Check sheet for the modelled part. Datum: model origin and axes. Units: mm. Coordinates: 2 decimals unless noted, no trailing zeros. Loops run counter-clockwise (first coordinate to the right, second up) from the corner with the lowest first, then second, coordinate; pieces in that order, holes last. Notation, with made-up numbers: M 84.25,73.5 L 104.25,73.5 A26 ccw 104.25,93.5 Z; hole C 23.5,-14 d9. An arc over 180 degrees is marked long. Use CSV: the item, a comma, the result in double quotes. Start each with the question number.
(1) Go/stop test with flat-tipped pins: pin 1 Ø1 at (x, z) = (-7, 1.5) entering from -Y; pin 2 Ø4 at (x, y) = (6.5, 0) entering from -Z; pin 3 Ø1 at (x, z) = (26.5, 1.5) entering from -Y. Record where each tip stops, or that it passes through.
(2) Section check C-C on x = -16.5. Record the cut outline in (y, z), and give its area (3 significant figures).
(3) Section check A-A on x = 6.5. Record the cut outline in (y, z) (3 decimals).
(4) Section check D-D on y = -27. Record the cut outline in (x, z), and give its area (3 significant figures).
(5) Section check B-B on z = 1.7. Record the cut outline in (x, y) (3 decimals), and give its area (3 significant figures).
(6) Scan lines: line 1 (Y direction, x = 6.5, z = 1.25) (3 decimals); line 2 (Y direction, x = 51, z = 0.3); line 3 (Y direction, x = -6.5, z = 1). Record each from-to range of solid material in increasing order.
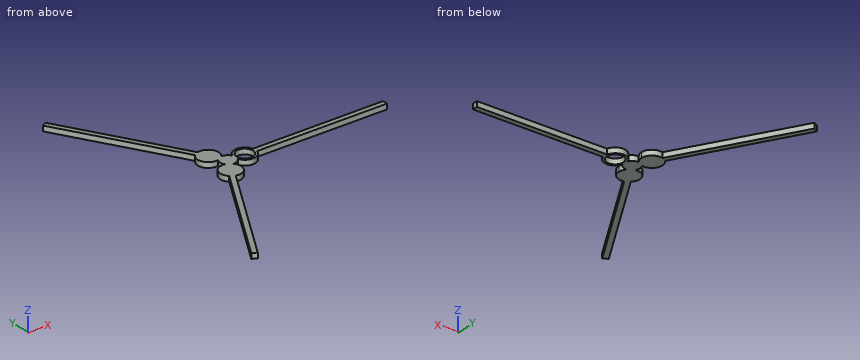
from build123d import *

# Parameters (mm, degrees)
F1_DEPTH = 2
F2_R     = 3.175
F3_DEPTH = 25


with BuildPart() as f1:
    # F0 (on Top) → F1 (new body)
    with BuildSketch(Plane.XY):
        with BuildLine():
            ThreePointArc((2.7115384615, -1.2835728151), (2.9269963601, -0.6577935145), (3, 0))
            ThreePointArc((3, 0), (2.9269963601, 0.6577935145), (2.7115384615, 1.2835728151))
            ThreePointArc((2.7115384615, 1.2835728151), (2.5, 0), (2.7115384615, -1.2835728151))
        make_face()
        with BuildLine():
            ThreePointArc((2.7115384615, -1.2835728151), (2.5, 0), (2.7115384615, 1.2835728151))
            ThreePointArc((2.7115384615, 1.2835728151), (1.5, 2.5980762114), (-0.2441625653, 2.9900475986))
            ThreePointArc((-0.2441625653, 2.9900475986), (-1.25, 2.1650635095), (-2.4673758962, 1.7064747835))
            ThreePointArc((-2.4673758962, 1.7064747835), (-3, 0), (-2.4673758962, -1.7064747835))
            ThreePointArc((-2.4673758962, -1.7064747835), (-1.25, -2.1650635095), (-0.2441625653, -2.9900475986))
            ThreePointArc((-0.2441625653, -2.9900475986), (1.5, -2.5980762114), (2.7115384615, -1.2835728151))
        make_face()
        with BuildLine():
            ThreePointArc((-2.4673758962, 1.7064747835), (-1.5, 2.5980762114), (-0.2441625653, 2.9900475986))
            ThreePointArc((-0.2441625653, 2.9900475986), (0.4932171817, 4.2190852933), (0.75, 5.6291651246))
            ThreePointArc((0.75, 5.6291651246), (-0.8294489344, 8.8136482127), (-4.3204662693, 9.4832670908))
            Line((-4.3204662693, 9.4832670908), (-6.0525170769, 8.4832670908))
            ThreePointArc((-6.0525170769, 8.4832670908), (-6.7857064923, 3.7586626253), (-2.4673758962, 1.7064747835))
        make_face()
        with BuildLine():
            ThreePointArc((-2.4673758962, 1.7064747835), (-1.25, 2.1650635095), (-0.2441625653, 2.9900475986))
            ThreePointArc((-0.2441625653, 2.9900475986), (-1.5, 2.5980762114), (-2.4673758962, 1.7064747835))
        make_face()
        with BuildLine():
            ThreePointArc((-2.4673758962, -1.7064747835), (-1.5, -2.5980762114), (-0.2441625653, -2.9900475986))
            ThreePointArc((-0.2441625653, -2.9900475986), (-1.25, -2.1650635095), (-2.4673758962, -1.7064747835))
        make_face()
        with BuildLine():
            ThreePointArc((0.75, -5.6291651246), (0.4932171817, -4.2190852933), (-0.2441625653, -2.9900475986))
            ThreePointArc((-0.2441625653, -2.9900475986), (-1.5, -2.5980762114), (-2.4673758962, -1.7064747835))
            ThreePointArc((-2.4673758962, -1.7064747835), (-6.7857064923, -3.7586626253), (-6.0525170769, -8.4832670908))
            Line((-6.0525170769, -8.4832670908), (-4.3204662693, -9.4832670908))
            ThreePointArc((-4.3204662693, -9.4832670908), (-0.8294489344, -8.8136482127), (0.75, -5.6291651246))
        make_face()
        with BuildLine():
            ThreePointArc((2.7115384615, 1.2835728151), (2.9269963601, 0.6577935145), (3, 0))
            ThreePointArc((3, 0), (2.9269963601, -0.6577935145), (2.7115384615, -1.2835728151))
            ThreePointArc((2.7115384615, -1.2835728151), (6.6479505639, -3.9972628924), (10.3729833462, -1))
            Line((10.3729833462, -1), (10.3729833462, 1))
            ThreePointArc((10.3729833462, 1), (6.6479505639, 3.9972628924), (2.7115384615, 1.2835728151))
        make_face()
        with BuildLine():
            Line((60.3729833462, 1), (10.3729833462, 1))
            ThreePointArc((10.3729833462, 1), (10.4681187851, 0.5040171699), (10.5, 0))
            ThreePointArc((10.5, 0), (10.4681187851, -0.5040171699), (10.3729833462, -1))
            Line((10.3729833462, -1), (60.3729833462, -1))
            Line((60.3729833462, -1), (60.3729833462, 1))
        make_face()
        with BuildLine():
            ThreePointArc((10.5, 0), (10.4681187851, 0.5040171699), (10.3729833462, 1))
            Line((10.3729833462, 1), (10.3729833462, -1))
            ThreePointArc((10.3729833462, -1), (10.4681187851, -0.5040171699), (10.5, 0))
        make_face()
        with BuildLine():
            Line((-4.3204662693, -9.4832670908), (-6.0525170769, -8.4832670908))
            ThreePointArc((-6.0525170769, -8.4832670908), (-5.25, -9.0932667397), (-4.3204662693, -9.4832670908))
        make_face()
        with BuildLine():
            ThreePointArc((-4.3204662693, -9.4832670908), (-5.25, -9.0932667397), (-6.0525170769, -8.4832670908))
            Line((-6.0525170769, -8.4832670908), (-31.0525170769, -51.7845372801))
            Line((-31.0525170769, -51.7845372801), (-29.3204662693, -52.7845372801))
            Line((-29.3204662693, -52.7845372801), (-4.3204662693, -9.4832670908))
        make_face()
        with BuildLine():
            ThreePointArc((-4.3204662693, 9.4832670908), (-5.25, 9.0932667397), (-6.0525170769, 8.4832670908))
            Line((-6.0525170769, 8.4832670908), (-4.3204662693, 9.4832670908))
        make_face()
        with BuildLine():
            Line((-31.0525170769, 51.7845372801), (-6.0525170769, 8.4832670908))
            ThreePointArc((-6.0525170769, 8.4832670908), (-5.25, 9.0932667397), (-4.3204662693, 9.4832670908))
            Line((-4.3204662693, 9.4832670908), (-29.3204662693, 52.7845372801))
            Line((-29.3204662693, 52.7845372801), (-31.0525170769, 51.7845372801))
        make_face()
    extrude(amount=F1_DEPTH)

    # F2 (on face) → F3 (cut)
    with BuildSketch(Plane.XY.offset(2)):
        with Locations((6.5, 0)):
            Circle(F2_R)
    extrude(amount=-F3_DEPTH, mode=Mode.SUBTRACT)


solid = f1.part
Outcome:
1,pin 1,"stops at y = -14.99"
1,pin 2,"passes through"
1,pin 3,"stops at y = -1"
2,outline,"M -30.58,0 L -26.58,0 L -26.58,2 L -30.58,2 Z; M 26.58,0 L 30.58,0 L 30.58,2 L 26.58,2 Z"
2,area,"16.0 mm²"
3,outline,"M -4,0 L -3.175,0 L -3.175,2 L -4,2 Z; M 3.175,0 L 4,0 L 4,2 L 3.175,2 Z"
4,outline,"M -16.74,0 L -14.43,0 L -14.43,2 L -16.74,2 Z"
4,area,"4.62 mm²"
5,outline,"M -31.053,-51.785 L -29.32,-52.785 L -4.32,-9.483 A4 ccw -0.244,-2.99 A3 ccw 2.712,-1.284 A4 ccw 10.373,-1 L 60.373,-1 L 60.373,1 L 10.373,1 A4 ccw 2.712,1.284 A3 ccw -0.244,2.99 A4 ccw -4.32,9.483 L -29.32,52.785 L -31.053,51.785 L -6.053,8.483 A4 ccw -2.467,1.706 A3 ccw -2.467,-1.706 A4 ccw -6.053,-8.483 Z; hole C 6.5,0 d6.35"
5,area,"444 mm²"
6,line 1,"y = -4 to -3.175, 3.175 to 4"
6,line 2,"y = -1 to 1"
6,line 3,"y = -13.26 to -9.26, -7.96 to -3.3, 3.3 to 7.96, 9.26 to 13.26"
